For this review, take the finished solid that the model builds, in its own axes (mm). Face numbers are marked on the shaded views. A direction names the side the tool comes from. Round coordinates to 2 decimals unless told otherwise and drop trailing zeros. Write each loop counter-clockwise with the first axis right and the second up, starting at its lowest first coordinate (ties: lowest second). Pieces come first, ordered by that corner, then holes. Notation, with made-up numbers: (79, 76.25) -> (128, 76.25) arc R26 cw to (128, 104.25) -> close; hole circle Ø6 at (-18, 18.5). An arc over 180 degrees is marked (long way). Answer in a Markdown table with one row per item.
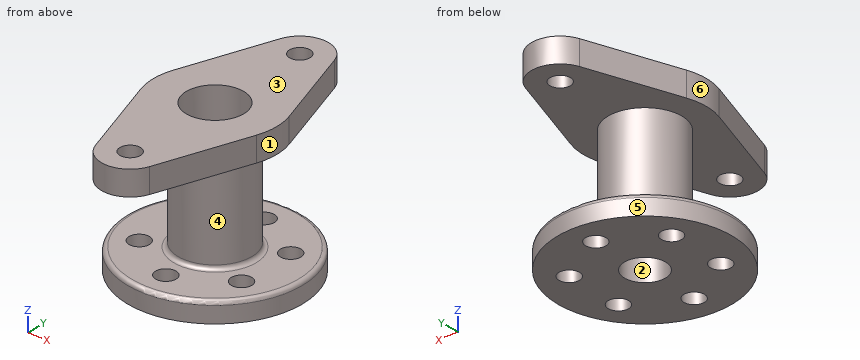
from build123d import *

# Parameters (mm, degrees)
SKETCH1_R                                          = 42.5
BOSS_EXTRUDE1_DEPTH                                = 10
SKETCH2_R                                          = 5
CUT_EXTRUDE1_DEPTH                                 = 61.930288035
CIRPATTERN2_COUNT                                  = 6
SKETCH3_R                                          = 18
BOSS_EXTRUDE2_DEPTH                                = 50
BOSS_EXTRUDE3_DEPTH                                = 12
SKETCH5_R                                          = 5
CUT_EXTRUDE3_DEPTH                                 = 106.291262695
CBORE_FOR_M2_5_PAN_HEAD_MACHINE_SCREW1_D           = 20
CBORE_FOR_M2_5_PAN_HEAD_MACHINE_SCREW1_CBORE_D     = 28
CBORE_FOR_M2_5_PAN_HEAD_MACHINE_SCREW1_CBORE_DEPTH = 25
FILLET1_R                                          = 2


with BuildPart() as part:
    # Sketch1 → Boss-Extrude1 (new body)
    with BuildSketch(Plane.XY):
        Circle(SKETCH1_R)
    extrude(amount=BOSS_EXTRUDE1_DEPTH)

    # Sketch2 → Cut-Extrude1 (cut, through all)
    with BuildSketch(Plane.XY.offset(10)):
        with Locations((0, 29)):
            Circle(SKETCH2_R)
    cut_extrude1 = extrude(amount=-CUT_EXTRUDE1_DEPTH, mode=Mode.SUBTRACT)

    # CirPattern2: Cut-Extrude1 ×6 about axis
    cirpattern2_axis = Axis((0, 0, 0), (0, 0, 1))
    for i in range(1, CIRPATTERN2_COUNT):
        add(cut_extrude1.rotate(cirpattern2_axis, i * 360 / CIRPATTERN2_COUNT), mode=Mode.SUBTRACT)

    # Sketch3 → Boss-Extrude2 (add)
    with BuildSketch(Plane.XY.offset(10)):
        Circle(SKETCH3_R)
    extrude(amount=BOSS_EXTRUDE2_DEPTH)

    # Sketch4 → Boss-Extrude3 (add)
    with BuildSketch(Plane.XY.offset(60)):
        with BuildLine():
            Line((-13.263845596, 54.48), (-28.422526278, 9.6))
            ThreePointArc((-28.422526278, 9.6), (-30, 0), (-28.422526278, -9.6))
            Line((-28.422526278, -9.6), (-13.263845596, -54.48))
            ThreePointArc((-13.263845596, -54.48), (0, -64), (13.263845596, -54.48))
            Line((13.263845596, -54.48), (28.422526278, -9.6))
            ThreePointArc((28.422526278, -9.6), (30, 0), (28.422526278, 9.6))
            Line((28.422526278, 9.6), (13.263845596, 54.48))
            ThreePointArc((13.263845596, 54.48), (0, 64), (-13.263845596, 54.48))
        make_face()
    extrude(amount=BOSS_EXTRUDE3_DEPTH)

    # Sketch5 → Cut-Extrude3 (cut, through all)
    with BuildSketch(Plane.XY.offset(72)):
        with Locations((0, 50)):
            Circle(SKETCH5_R)
    cut_extrude3 = extrude(amount=-CUT_EXTRUDE3_DEPTH, mode=Mode.SUBTRACT)

    # Mirror1: Cut-Extrude3 across plane
    add(cut_extrude3.mirror(Plane.ZX), mode=Mode.SUBTRACT)

    # CBORE for M2.5 Pan Head Machine Screw1 (through all)
    with Locations(Plane.XY.offset(72)):
        with Locations((0, 0)):
            CounterBoreHole(CBORE_FOR_M2_5_PAN_HEAD_MACHINE_SCREW1_D / 2, CBORE_FOR_M2_5_PAN_HEAD_MACHINE_SCREW1_CBORE_D / 2, CBORE_FOR_M2_5_PAN_HEAD_MACHINE_SCREW1_CBORE_DEPTH)

    # Fillet1
    fillet1_edges = [part.edges().sort_by_distance(p)[0] for p in [
        (-18, 0, 10),
        (-42.5, 0, 10),
    ]]
    fillet(fillet1_edges, radius=FILLET1_R)


solid = part.part
1) Consider section A-A on z = 66. State the section outline as (x, y) points, then the cut area to 3 significant figures.
Solved:
| item | result |
|---|---|
| outline | (-28.42, -9.6) -> (-13.26, -54.48) arc R14 ccw to (13.26, -54.48) -> (28.42, -9.6) arc R30 ccw to (28.42, 9.6) -> (13.26, 54.48) arc R14 ccw to (-13.26, 54.48) -> (-28.42, 9.6) arc R30 ccw to start; hole circle Ø28 at (0, 0); hole circle Ø10 at (0, -50); hole circle Ø10 at (0, 50) |
| area | 4,470 mm² |
2) Consider section B-B on y = 0. State the section outline as (x, z) points, then the cut area to 3 significant figures.
Solved:
| item | result |
|---|---|
| outline | (-42.5, 0) -> (-10, 0) -> (-10, 47) -> (-14, 47) -> (-14, 72) -> (-30, 72) -> (-30, 60) -> (-18, 60) -> (-18, 12) arc R2 cw to (-20, 10) -> (-40.5, 10) arc R2 ccw to (-42.5, 8) -> close; (10, 0) -> (42.5, 0) -> (42.5, 8) arc R2 ccw to (40.5, 10) -> (20, 10) arc R2 cw to (18, 12) -> (18, 60) -> (30, 60) -> (30, 72) -> (14, 72) -> (14, 47) -> (10, 47) -> close |
| area | 1,730 mm² |
3) Consider section C-C on z = 22. State the section outline as (x, y) points, then the cut area to 3 significant figures.
Solved:
| item | result |
|---|---|
| outline | circle Ø36 at (0, 0); hole circle Ø20 at (0, 0) |
| area | 704 mm² |
4) For the marked faces 4, 5 and 6, list the 3-axis set-ups (+Z, -Z, +X, -X, +Y, -Y) from which the entire face can be reached by the end or side of a thin tool; tool diameter is ignored.
Solved:
| item | result |
|---|---|
| face 4 | none |
| face 5 | -Z |
| face 6 | +Z, -X |
5) Clearance check with flat-ended pins moving along their axes: pin 1 Ø6 at (x, y) = (0, 29) entering from -Z; pin 2 Ø12 at (y, z) = (-15.5, 11) entering from -X; pin 3 Ø13 at (x, y) = (25.11, 14.5) entering from -Z; pin 4 Ø5 at (y, z) = (-6.5, 46.5) entering from -X. State where each tip first meets the part, or that it passes through.
Solved:
| item | result |
|---|---|
| pin 1 | z = 60 |
| pin 2 | x = -41.25 |
| pin 3 | z = 0 |
| pin 4 | x = -17.55 |
6) For line 1 (Z direction, x = 24.5, y = 9); line 2 (Y direction, x = 0, z = 55); line 3 (Z direction, x = -33.5, y = 15), list the stretches that pass through material, from the lowest coordinate up. Write a range as [from, to].
Solved:
| item | result |
|---|---|
| line 1 | [0, 10], [60, 72] |
| line 2 | [-18, -14], [14, 18] |
| line 3 | [0, 10] |
7) Consider section D-D on x = 0. State how many separate pieces and enclosed holes the cut face has, then the cut area to 3 significant figures.
Solved:
| item | result |
|---|---|
| separate pieces | 6 |
| enclosed holes | 0 |
| area | 2,110 mm² |
8) Mouldability with a two-part tool opening along Y and no side actions: class the marked faces 1, 2 and 3 as pulls with the +Y half, pulls with the -Y half, needs draft (parallel to the pull), parting line crosses it, or undercut.
Solved:
| item | result |
|---|---|
| face 1 | parting line crosses it |
| face 2 | undercut |
| face 3 | needs draft |
